Here's how the part is built. I have some questions about the finished solid (model axes, mm). A direction names the side the tool comes from. Round coordinates to 2 decimals unless told otherwise and drop trailing zeros. Write each loop counter-clockwise with the first axis right and the second up, starting at its lowest first coordinate (ties: lowest second). Pieces come first, ordered by that corner, then holes. Notation, with made-up numbers: (31.25, 78.5) -> (49.25, 78.5) arc R17 ccw to (49.25, 98.5) -> close; hole circle Ø10 at (13.5, 74). An arc over 180 degrees is marked (long way). Put each result on its own line as item: value. Start each with the question number.
1) Will these pins go through, and if not, where does the flat tip stop? P1, Ø2, axis at x = 0, y = -4, coming from the -Z side; P2, Ø1.5, axis at x = -1, y = -8.5, coming from the -Z side; P3, Ø1.1, axis at x = -0.5, y = 5.5, coming from the -Z side.
2) If I drill on line 1 along Y through (x, z) = (0.65, -1.55); line 2 along X through (y, z) = (0, 0); line 3 along X through (y, z) = (2, 1), over which ranges is the centre line in solid material (lowest first)? Write a range as [from, to].
3) I want a section at B-B, the plane z = 0. List the corners of the cut face in (x, y) for me, then the cut area to 3 significant figures.
4) Which directions (+Z, -Z, +X, -X, +Y, -Y) give clear straight access to the entire face, cutting with the end or side of a thin tool? Please do faces 1 (the flat face through (0, -26, -1)), 2 (the flat face through (0, -1, -1)), 3 (the cylindrical face through (0.04, 4.43, 1.25)), 4 (the cylindrical face through (0, -24.8, 1.5)).
5) I want a section at A-A, the plane x = 0. List the corners of the cut face in (y, z) for me.
6) I want a section at C-C, the plane y = -0.5. List the corners of the cut face in (x, z) for me.
from build123d import *

# Parameters (mm, degrees)
CUT_EXTRUDE_3_REACH = 38.898
CUT_EXTRUDE_START   = -10.35
CUT_EXTRUDE_5_DEPTH = 10.35
CUT_EXTRUDE_7_DEPTH = 1.4


with BuildPart() as part:
    # 草图1 → 旋转2 (revolve)
    with BuildSketch(Plane.XY, mode=Mode.PRIVATE) as revolve_2_sk:
        Polygon((1.25, 5.955283348), (0, 5.955283348), (0, -30.844716652), (1.25, -30.844716652), (1.25, -29.144716652), (1.5, -29.144716652), (1.5, -20.494716652), (1.9, -20.494716652), (1.9, -5.794716652), (1.5, -5.794716652), (1.5, 2.855283348), (1.25, 2.855283348), align=None)
    revolve(revolve_2_sk.sketch.rotate(Axis((0, 5.955283348, 0), (0, -1, 0)), 180), axis=Axis((0, 5.955283348, 0), (0, -1, 0)))

    # 切除-拉伸3: up to this face of the body (flat: up to its plane)
    cut_extrude_3_end = Plane(part.part.faces().sort_by_distance((1.846259885, -5.794716652, 0))[0])
    # 草图5 → 切除-拉伸3 (cut, up to the picked face)
    with BuildSketch(Plane(origin=(0, 5.955283348, 0), x_dir=(1, 0, 0), z_dir=(0, 1, 0)), mode=Mode.PRIVATE) as cut_extrude_3_sk1:
        with BuildLine():
            Line((-1.118033989, 1), (1.118033989, 1))
            ThreePointArc((1.118033989, 1), (0, 1.5), (-1.118033989, 1))
        make_face()
    cut_extrude_3_tool1 = split(extrude(cut_extrude_3_sk1.sketch, amount=-CUT_EXTRUDE_3_REACH, mode=Mode.PRIVATE), bisect_by=cut_extrude_3_end, keep=Keep.BOTH, mode=Mode.PRIVATE)
    add(cut_extrude_3_tool1.solids().sort_by(Axis((0, 5.955283, -1.203164), (0, -1, 0)))[0], mode=Mode.SUBTRACT)

    # 草图7 → 切除-拉伸5 (cut)
    with BuildSketch(Plane.XZ.offset(30.844716652).offset(CUT_EXTRUDE_START)):
        with BuildLine():
            Line((1.118033989, -1), (-1.118033989, -1))
            ThreePointArc((-1.118033989, -1), (0, -1.5), (1.118033989, -1))
        make_face()
    extrude(amount=CUT_EXTRUDE_5_DEPTH, mode=Mode.SUBTRACT)

    # 草图10 → 切除-拉伸7 (cut)
    with BuildSketch(Plane(origin=(0, 5.955283348, 0), x_dir=(1, 0, 0), z_dir=(0, 1, 0))):
        with BuildLine():
            Line((-1, 0.75), (1, 0.75))
            ThreePointArc((1, 0.75), (0, 1.25), (-1, 0.75))
        make_face()
    extrude(amount=-CUT_EXTRUDE_7_DEPTH, mode=Mode.SUBTRACT)


solid = part.part
Findings:
1. P1: stops at z = -1
1. P2: stops at z = -1.88
1. P3: stops at z = -0.75
2. line 1: y = [-20.49, -5.79]
2. line 2: x = [-1.5, 1.5]
2. line 3: x = [-1.12, 1.12]
3. outline: (-1.9, -20.49) -> (-1.5, -20.49) -> (-1.5, -29.14) -> (-1.25, -29.14) -> (-1.25, -30.84) -> (1.25, -30.84) -> (1.25, -29.14) -> (1.5, -29.14) -> (1.5, -20.49) -> (1.9, -20.49) -> (1.9, -5.79) -> (1.5, -5.79) -> (1.5, 2.86) -> (1.25, 2.86) -> (1.25, 5.96) -> (-1.25, 5.96) -> (-1.25, 2.86) -> (-1.5, 2.86) -> (-1.5, -5.79) -> (-1.9, -5.79) -> close
3. area: 120 mm2
4. face 1: -Z, +X, -X, -Y
4. face 2: -Z, +X, -X, +Y
4. face 3: +Y
4. face 4: -Y
5. outline: (-30.84, -1) -> (-20.49, -1) -> (-20.49, -1.9) -> (-5.79, -1.9) -> (-5.79, -1) -> (4.56, -1) -> (4.56, -0.75) -> (5.96, -0.75) -> (5.96, 1.25) -> (2.86, 1.25) -> (2.86, 1.5) -> (-5.79, 1.5) -> (-5.79, 1.9) -> (-20.49, 1.9) -> (-20.49, 1.5) -> (-29.14, 1.5) -> (-29.14, 1.25) -> (-30.84, 1.25) -> close
6. outline: (-1.12, -1) -> (1.12, -1) arc R1.5 ccw (long way) to start
